Source: CAD feature listing. Evaluate the final solid. Frame: model axes, mm. A direction names the side the tool comes from. Give positions to 0.01 mm unless a question says otherwise; leave off trailing zeros. Order: outer loops, then holes, each group sorted by start corner. A loop starts at its lowest first (then second) coordinate and runs counter-clockwise, first axis right, second up. Notation, with made-up numbers: M 33,21.25 L 82,21.25 A20 cw 82,59.25 Z; hole C 76,-8.5 d7. An arc over 180 degrees is marked long. Return JSON: item names as keys, results as strings.
from build123d import *

# Parameters (mm, degrees)
F1_DEPTH = 63.5
F2_DEPTH = 25.4
F3_DEPTH = 7.9375
F0_W     = 25.4
F0_H     = 28.575
F5_R     = 6.35


with BuildPart() as f1:
    # F0 (on Front) → F1 (new body, symmetric)
    with BuildSketch(Plane.XZ):
        Polygon((41.275, -9.525), (41.275, 9.525), (22.225, 9.525), (-41.275, 9.525), (-41.275, -9.525), align=None)
    extrude(amount=F1_DEPTH, both=True)

    # F0 (on Front) → F2 (join, symmetric)
    with BuildSketch(Plane.XZ):
        with BuildLine():
            Line((22.225, 9.525), (41.275, 9.525))
            Line((41.275, 9.525), (41.275, 27.0002))
            ThreePointArc((41.275, 27.0002), (45.92468, 38.22552), (57.15, 42.8752))
            Line((57.15, 42.8752), (60.325, 42.8752))
            Line((60.325, 42.8752), (60.325, 61.9252))
            Line((60.325, 61.9252), (57.15, 61.9252))
            add(Edge.make_bspline(
                [(55.397646, 61.88121), (55.98511, 61.899276), (56.569297, 61.913923), (57.15, 61.9252)],
                knots=[109.698867, 109.698867, 109.698867, 109.698867, 111.504536, 111.504536, 111.504536, 111.504536], degree=3))
            ThreePointArc((55.397646, 61.88121), (31.842327, 51.068381), (22.225, 27.0002))
            Line((22.225, 27.0002), (22.225, 9.525))
        make_face()
        Polygon((60.325, 61.9252), (60.325, 42.8752), (60.325, 38.1), (85.725, 38.1), (85.725, 66.675), (60.325, 66.675), align=None)
    extrude(amount=F2_DEPTH, both=True)

    # F0 (on Front) → F3 (join, symmetric)
    with BuildSketch(Plane.XZ):
        with BuildLine():
            Line((-41.275, 9.525), (22.225, 9.525))
            Line((22.225, 9.525), (22.225, 27.0002))
            ThreePointArc((22.225, 27.0002), (31.842327, 51.068381), (55.397646, 61.88121))
            add(Edge.make_bspline(
                [(-41.275, 9.525), (-28.07554, 47.064815), (19.707757, 60.783645), (55.397646, 61.88121)],
                knots=[0, 0, 0, 0, 109.698867, 109.698867, 109.698867, 109.698867], degree=3))
        make_face()
    extrude(amount=F3_DEPTH, both=True)

    # F0 (on Front) → F4 (revolve)
    with BuildSketch(Plane.XZ):
        with Locations((98.425, 52.3875)):
            Rectangle(F0_W, F0_H)
    revolve(axis=Axis((85.725, 0, 52.3875), (0, 0, 1)))

    # F5
    f5_edges = [f1.edges().sort_by_distance(p)[0] for p in [
        (-41.275, -63.5, 0),
        (41.275, -63.5, 0),
        (41.275, 63.5, 0),
        (-41.275, 63.5, 0),
    ]]
    fillet(f5_edges, radius=F5_R)


solid = f1.part
1. Section query B-B (y = -36.5). Return loops of the section in (x, z) (3 decimals), then the cut area to 3 significant figures.
Evaluation:
{"outline": "M -41.275,-9.525 L 41.275,-9.525 L 41.275,9.525 L -41.275,9.525 Z", "area": "1,570 mm^2"}
2. Section query A-A (x = 69). Return loops of the section in (y, z) (3 decimals).
Evaluation:
{"outline": "M -25.4,38.1 L 25.4,38.1 L 25.4,66.675 L -25.4,66.675 Z"}
3. Set-up query: faces 4 (the face through (-4, -7.938, 30)), 5 (the face through (86, 0, 38.1)), 6 (the face through (22.225, 17, 18)), 7 (the face through (54, 25.4, 45)). Return all of +Z, -Z, +X, -X, +Y, -Y with unobstructed straight access to the full face (end or side cutting, diameter ignored); none if empty.
Evaluation:
{"face 4": "+Z, -X, -Y", "face 5": "-Z, +X, +Y, -Y", "face 6": "+Z, -X, +Y", "face 7": "+Z, +X, -X, +Y"}
4. First-contact query: pin 1 (2.5 mm diameter, centred on y = 6.5, z = 65.5, fed in from -X) (3 decimals); pin 2 (17 mm diameter, centred on x = 42, z = 36, fed in from -Y); pin 3 (15.5 mm diameter, centred on x = -2, z = 48.5, fed in from +Y). Flat tips, straight axial feed; report the tip coordinate or a pass-through.
Evaluation:
{"pin 1": "stops at x = 60.325", "pin 2": "stops at y = -25.4", "pin 3": "stops at y = 7.94"}
5. Ray query, probe 1 along Z at (x, y) = (2.5, -51) (3 decimals); probe 2 along Z at (x, y) = (99, 5.5) (3 decimals); probe 3 along X at (y, z) = (-47.5, 0.5) (3 decimals). Return the intervals inside material, ascending.
Evaluation:
{"probe 1": "z = -9.525 to 9.525", "probe 2": "z = 38.1 to 66.675", "probe 3": "x = -41.275 to 41.275"}
6. Draft query along X for faces 1 (the face through (54, -25.4, 45)), 2 (the face through (60.325, 0, 41)), 3 (the face through (32.1, -16.791, 51.336)). Return one class per face: pulls with the +X half, pulls with the -X half, needs draft (parallel to the pull), parting line crosses it, or undercut.
Evaluation:
{"face 1": "needs draft", "face 2": "undercut", "face 3": "pulls with the -X half"}
